The model under review builds one solid part; all positions refer to its coordinate system, in mm. Face numbers are marked on the shaded views. A direction names the side the tool comes from. Round coordinates to 2 decimals unless told otherwise and drop trailing zeros. Order: outer loops, then holes, each group sorted by start corner. A loop starts at its lowest first (then second) coordinate and runs counter-clockwise, first axis right, second up. Notation, with made-up numbers: M -31.75,-14.5 L -27.75,-14.5 A13 ccw -27.75,-3.5 Z; hole C -36,15.25 d9. An arc over 180 degrees is marked long. Answer as CSV lines item,"result". Start each with the question number.
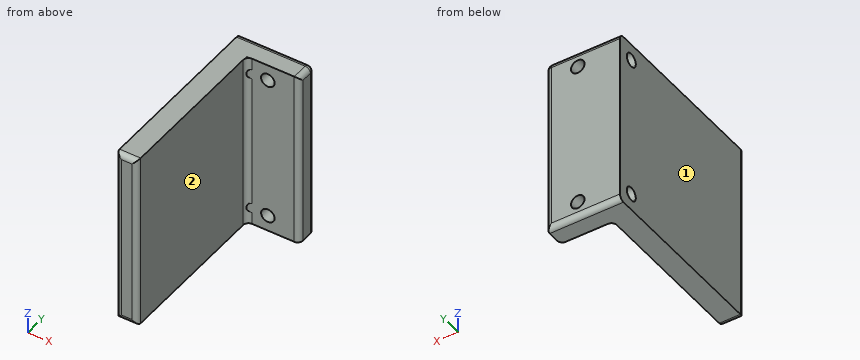
from build123d import *

# Parameters (mm, degrees)
SKETCH1_W           = 429.768
SKETCH1_H           = 448.056
SKETCH1_R           = 16.256
BOSS_EXTRUDE1_DEPTH = 50.8
SKETCH2_W           = 429.768
SKETCH2_H           = 52.07
BOSS_EXTRUDE2_DEPTH = 127
SKETCH3_R           = 16.256
CUT_EXTRUDE1_DEPTH  = 76.2
FILLET1_R           = 12.7


with BuildPart() as part:
    # Sketch1 → Boss-Extrude1 (new body)
    with BuildSketch(Plane(origin=(0, 0, 0), x_dir=(0, 0, -1), z_dir=(1, 0, 0))):
        Rectangle(SKETCH1_W, SKETCH1_H)
        with Locations((-173.99, 183.134)):
            Circle(SKETCH1_R, mode=Mode.SUBTRACT)
        with Locations((173.99, 183.134)):
            Circle(SKETCH1_R, mode=Mode.SUBTRACT)
    extrude(amount=BOSS_EXTRUDE1_DEPTH)

    # Sketch2 → Boss-Extrude2 (add)
    with BuildSketch(Plane(origin=(50.8, 0, 0), x_dir=(0, 0, -1), z_dir=(1, 0, 0))):
        with Locations((0, 197.993)):
            Rectangle(SKETCH2_W, SKETCH2_H)
    extrude(amount=BOSS_EXTRUDE2_DEPTH)

    # Sketch3 → Cut-Extrude1 (cut)
    with BuildSketch(Plane(origin=(0, 224.028, 0), x_dir=(1, 0, 0), z_dir=(0, 1, 0))):
        with Locations(Location((101.6, 176.012040492, 0), (0, 0, 270))):
            Circle(SKETCH3_R)
        with Locations(Location((101.6, -176.012040492, 0), (0, 0, 270))):
            Circle(SKETCH3_R)
    extrude(amount=-CUT_EXTRUDE1_DEPTH, mode=Mode.SUBTRACT)

    # Fillet1
    # the kernel refuses this fillet: 12.7 mm, written as the material it adds along each edge
    with BuildSketch(Plane(origin=(50.8, 171.958, -214.884), x_dir=(0, -1, 0), z_dir=(0, 0, 1))) as fillet1_piece_1_section:
        with BuildLine():
            CenterArc((FILLET1_R, FILLET1_R), FILLET1_R, 180, 90)
            Line((0, FILLET1_R), (0, 0))
            Line((0, 0), (FILLET1_R, 0))
        make_face()
    fillet1_piece_1 = extrude(amount=60.839146761, mode=Mode.PRIVATE)
    fillet1_piece_1 = fillet1_piece_1 - Plane(origin=(53.390848129, 183.134, -173.99), x_dir=(0, 0, -1), z_dir=(-1, 0, 0)) * Cylinder(16.256, 173, mode=Mode.PRIVATE)
    add(fillet1_piece_1)
    with BuildSketch(Plane(origin=(50.8, 171.958, -193.935146761), x_dir=(0, -1, 0), z_dir=(0, 0, 1))) as fillet1_piece_2_section:
        with BuildLine():
            CenterArc((FILLET1_R, FILLET1_R), FILLET1_R, 180, 90)
            Line((0, FILLET1_R), (0, 0))
            Line((0, 0), (FILLET1_R, 0))
        make_face()
    fillet1_piece_2 = extrude(amount=387.870293522, mode=Mode.PRIVATE)
    fillet1_piece_2 = fillet1_piece_2 - Plane(origin=(53.573862422, 183.134, 173.99), x_dir=(0, 0, -1), z_dir=(-1, 0, 0)) * Cylinder(16.256, 827, mode=Mode.PRIVATE)
    fillet1_piece_2 = fillet1_piece_2 - Plane(origin=(53.573862422, 183.134, -173.99), x_dir=(0, 0, -1), z_dir=(-1, 0, 0)) * Cylinder(16.256, 827, mode=Mode.PRIVATE)
    add(fillet1_piece_2)
    with BuildSketch(Plane(origin=(50.8, 171.958, 154.044853239), x_dir=(0, -1, 0), z_dir=(0, 0, 1))) as fillet1_piece_3_section:
        with BuildLine():
            CenterArc((FILLET1_R, FILLET1_R), FILLET1_R, 180, 90)
            Line((0, FILLET1_R), (0, 0))
            Line((0, 0), (FILLET1_R, 0))
        make_face()
    fillet1_piece_3 = extrude(amount=60.839146761, mode=Mode.PRIVATE)
    fillet1_piece_3 = fillet1_piece_3 - Plane(origin=(53.390848027, 183.134, 173.99), x_dir=(0, 0, -1), z_dir=(-1, 0, 0)) * Cylinder(16.256, 173, mode=Mode.PRIVATE)
    add(fillet1_piece_3)
    # the kernel refuses this fillet: 12.7 mm, written as the material it takes off along each edge
    with BuildSketch(Plane(origin=(165.1, 211.328, 202.184), x_dir=(1, 0, 0), z_dir=(0, 1, 0))) as fillet1_2_piece_1_section:
        Polygon((0, 0), (FILLET1_R * 1.02, 0), (FILLET1_R * 1.02, -FILLET1_R * 1.02), (0, -FILLET1_R * 1.02), align=None)
    fillet1_2_piece_1 = extrude(amount=FILLET1_R * 1.02, mode=Mode.PRIVATE)
    fillet1_2_piece_1 = fillet1_2_piece_1 - Plane(origin=(165.1, 211.328, 202.184), x_dir=(-0.7071067811865475, 0, -0.7071067811865475), z_dir=(0, 1, 0)) * Sphere(FILLET1_R, mode=Mode.PRIVATE)
    add(fillet1_2_piece_1, mode=Mode.SUBTRACT)
    with BuildSketch(Plane(origin=(-31.75, -224.028, -214.884), x_dir=(0, 0, 1), z_dir=(1, 0, 0))) as fillet1_2_piece_2:
        with BuildLine():
            CenterArc((FILLET1_R, -FILLET1_R), FILLET1_R, 90, 90)
            Line((0, -FILLET1_R), (0, 0))
            Line((0, 0), (FILLET1_R, 0))
        make_face()
    extrude(amount=114.3, mode=Mode.SUBTRACT)
    with BuildSketch(Plane(origin=(-31.75, -224.028, 214.884), x_dir=(0, 0, -1), z_dir=(1, 0, 0))) as fillet1_2_piece_3:
        with BuildLine():
            CenterArc((FILLET1_R, FILLET1_R), FILLET1_R, 180, 90)
            Line((0, FILLET1_R), (0, 0))
            Line((0, 0), (FILLET1_R, 0))
        make_face()
    extrude(amount=114.3, mode=Mode.SUBTRACT)
    with BuildSketch(Plane(origin=(165.1, 224.028, 214.884), x_dir=(0, 0, -1), z_dir=(-1, 0, 0))) as fillet1_2_piece_4:
        with BuildLine():
            CenterArc((FILLET1_R, FILLET1_R), FILLET1_R, 180, 90)
            Line((0, FILLET1_R), (0, 0))
            Line((0, 0), (FILLET1_R, 0))
        make_face()
    extrude(amount=196.85, mode=Mode.SUBTRACT)
    with BuildSketch(Plane(origin=(-31.75, 224.028, -214.884), x_dir=(0, 0, 1), z_dir=(1, 0, 0))) as fillet1_2_piece_5:
        with BuildLine():
            CenterArc((FILLET1_R, FILLET1_R), FILLET1_R, 180, 90)
            Line((0, FILLET1_R), (0, 0))
            Line((0, 0), (FILLET1_R, 0))
        make_face()
    extrude(amount=241.3, mode=Mode.SUBTRACT)
    with BuildSketch(Plane(origin=(177.8, 140.208, 214.884), x_dir=(0, 0, -1), z_dir=(0, 1, 0))) as fillet1_2_piece_6:
        with BuildLine():
            CenterArc((FILLET1_R, FILLET1_R), FILLET1_R, 180, 90)
            Line((0, FILLET1_R), (0, 0))
            Line((0, 0), (FILLET1_R, 0))
        make_face()
    extrude(amount=71.12, mode=Mode.SUBTRACT)
    with BuildSketch(Plane(origin=(177.8, 171.958, -246.634), x_dir=(-1, 0, 0), z_dir=(0, 0, 1)), Plane(origin=(0, -224.028, 246.634), x_dir=(1, 0, 0), z_dir=(0, 0, -1))) as fillet1_2_piece_7:
        with BuildLine():
            CenterArc((FILLET1_R, -FILLET1_R), FILLET1_R, 90, 90)
            Line((0, -FILLET1_R), (0, 0))
            Line((0, 0), (FILLET1_R, 0))
        make_face()
    extrude(amount=493.268, mode=Mode.SUBTRACT)
    with BuildSketch(Plane(origin=(177.8, 224.028, 202.184), x_dir=(-1, 0, 0), z_dir=(0, 0, -1))) as fillet1_2_piece_8:
        with BuildLine():
            CenterArc((FILLET1_R, -FILLET1_R), FILLET1_R, 90, 90)
            Line((0, -FILLET1_R), (0, 0))
            Line((0, 0), (FILLET1_R, 0))
        make_face()
    extrude(amount=448.818, mode=Mode.SUBTRACT)
    with BuildSketch(Plane(origin=(50.8, -224.028, 246.634), x_dir=(-1, 0, 0), z_dir=(0, 0, -1))) as fillet1_2_piece_9:
        with BuildLine():
            CenterArc((FILLET1_R, FILLET1_R), FILLET1_R, 180, 90)
            Line((0, FILLET1_R), (0, 0))
            Line((0, 0), (FILLET1_R, 0))
        make_face()
    extrude(amount=493.268, mode=Mode.SUBTRACT)


solid = part.part
Item 1: Consider section C-C (z = -81). State the section outline as (x, y) points.
Item 2: Consider section D-D (x = 70). State the section outline as (y, z) points.
Item 3: Consider section A-A (x = 101.6). State the section outline as (y, z) points.
Item 4: Tool access review of the marked faces 1 and 2: name each direction out of +Z, -Z, +X, -X, +Y, -Y from which nothing blocks a thin tool from reaching the whole face with its end or side.
Item 5: Consider section B-B (z = 180.5). State the section outline as (x, y) points.
Item 6: For pin 1 (1.5 mm diameter, centred on y = -149.5, z = 78.5, fed in from +X); pin 2 (22 mm diameter, centred on y = 187, z = 175, fed in from -X), all flat-tipped, find the tip position at first contact; note any pin that passes through.
Item 7: Wall thickness on probe 1 along Y at (x, z) = (24.5, 173.99); probe 2 along Y at (x, z) = (144, -17); probe 3 along Y at (x, z) = (39, 58.5): over which ranges is each line inside the solid? List them lowest first. Write a range as [from, to].
Reported:
1,outline,"M 0,-211.33 A12.7 ccw 12.7,-224.03 L 38.1,-224.03 A12.7 ccw 50.8,-211.33 L 50.8,159.26 A12.7 cw 63.5,171.96 L 165.1,171.96 A12.7 ccw 177.8,184.66 L 177.8,211.33 A12.7 ccw 165.1,224.03 L 0,224.03 Z"
2,outline,"M 171.96,-214.88 L 211.33,-214.88 A12.7 ccw 224.03,-202.18 L 224.03,202.18 A12.7 ccw 211.33,214.88 L 171.96,214.88 Z"
3,outline,"M 171.96,-214.88 L 211.33,-214.88 A12.7 ccw 224.03,-202.18 L 224.03,-192.27 L 171.96,-192.27 Z; M 171.96,-159.76 L 224.03,-159.76 L 224.03,159.76 L 171.96,159.76 Z; M 171.96,192.27 L 224.03,192.27 L 224.03,202.18 A12.7 ccw 211.33,214.88 L 171.96,214.88 Z"
4,face 1,"+Z, -Z, -X, +Y, -Y"
4,face 2,"+Z, -Z, +X, -Y"
5,outline,"M 0,-211.33 A12.7 ccw 12.7,-224.03 L 38.1,-224.03 A12.7 ccw 50.8,-211.33 L 50.8,159.26 A12.7 cw 54.52,168.24 L 0,168.24 Z; M 0,198.03 L 50.8,198.03 L 50.8,171.96 L 85.98,171.96 L 85.98,224.03 L 0,224.03 Z; M 117.22,171.96 L 165.1,171.96 A12.7 ccw 177.8,184.66 L 177.8,211.33 A12.7 ccw 165.1,224.03 L 117.22,224.03 Z"
6,pin 1,"stops at x = 50.8"
6,pin 2,"stops at x = 50.8"
7,probe 1,"y = [-224.03, 166.88], [199.39, 224.03]"
7,probe 2,"y = [171.96, 224.03]"
7,probe 3,"y = [-224, 224.03]"
